Autodesk Fusion 360 part; units mm, degrees
sketch "スケッチ1" plane through (0, 0, 0) normal (0, 1, 0) x (1, 0, 0)
  circle A0 centre (0, 0) radius 14.8
  dimension "d1" = 29.6
extrude "押し出し1" add sketch "スケッチ1" along normal blind 10
sketch "スケッチ2" plane through (0, 10, 0) normal (0, 1, 0) x (-1, 0, 0)
  circle A0 centre (0, 0) radius 14.8
  circle A1 centre (0, 0) radius 16.5
  dimension "d4" = 33
extrude "押し出し2" add sketch "スケッチ2" along normal blind 19 contours A0 | A1
ref_plane "作業平面1" through (0, 24, 0) normal (0, 1, 0) x (-1, 0, 0)
sketch "スケッチ3" plane through (0, 24, 0) normal (0, 1, 0) x (1, 0, 0)
ref_plane "作業平面2" through (0, 29, 0) normal (0, -1, 0) x (-1, 0, 0)
sketch "スケッチ5" plane through (0, 29, 0) normal (0, -1, 0) x (1, 0, 0)
  circle A0 centre (0, 0) radius 19
  dimension "d12" = 38
extrude "押し出し4" add sketch "スケッチ5" against normal blind 2.5
sketch "スケッチ6" plane through (0, 29, 0) normal (0, -1, 0) x (1, 0, 0)
  circle A0 centre (0, 0) radius 18
  dimension "d15" = 36
extrude "押し出し5" add sketch "スケッチ6" along normal blind 2.2
ref_plane "作業平面4" through (0, 24.8, 0) normal (0, -1, 0) x (1, 0, 0)
CAD build for the part. Positions are in the model's coordinates, mm. A direction names the side the tool comes from. Round coordinates to 2 decimals unless told otherwise and drop trailing zeros. Write each loop counter-clockwise with the first axis right and the second up, starting at its lowest first coordinate (ties: lowest second). Pieces come first, ordered by that corner, then holes.
Item 1: Tool access for faces 1 (the cylindrical face through (8.767, 30.232, -16.856)), 2 (the flat face through (8, 26.8, -15)): list every direction of +Z, -Z, +X, -X, +Y, -Y with a clear straight run to the whole face (end or side of a thin tool).
Filled in:
face 1: +Y, -Y
face 2: -Y
Item 2: Band-saw the part on B-B on x = 0. Write the cut outline in (y, z), then the cut area to 3 significant figures.
Filled in:
outline: (0, -14.8) - (10, -14.8) - (10, -16.5) - (26.8, -16.5) - (26.8, -18) - (29, -18) - (29, -19) - (31.5, -19) - (31.5, 19) - (29, 19) - (29, 18) - (26.8, 18) - (26.8, 16.5) - (10, 16.5) - (10, 14.8) - (0, 14.8) - close
area: 1,020 mm2
Item 3: Band-saw the part on C-C on y = 4.5. Write the cut outline in (x, z).
Filled in:
outline: circle Ø29.6 at (0, 0)
Item 4: Drop flat-ended pins along their axis: pin 1 Ø5 at (x, y) = (-11, 4.5) entering from +Z; pin 2 Ø5 at (y, z) = (6, 3.5) entering from +X; pin 3 Ø8 at (y, z) = (13, -10) entering from -X. Give the stop position or say it passes through.
Filled in:
pin 1: stops at z = 12.12
pin 2: stops at x = 14.77
pin 3: stops at x = -15.37
Item 5: Band-saw the part on A-A on z = 0. Write the cut outline in (x, y).
Filled in:
outline: (-19, 29) - (-18, 29) - (-18, 26.8) - (-16.5, 26.8) - (-16.5, 10) - (-14.8, 10) - (-14.8, 0) - (14.8, 0) - (14.8, 10) - (16.5, 10) - (16.5, 26.8) - (18, 26.8) - (18, 29) - (19, 29) - (19, 31.5) - (-19, 31.5) - close
Item 6: Band-saw the part on D-D on y = 13.5. Write the cut outline in (x, z), then the cut area to 3 significant figures.
Filled in:
outline: circle Ø33 at (0, 0)
area: 855 mm2
Item 7: Drill centre lines: L1, parallel to Y at x = 0, z = -15.5; L2, parallel to X at y = 2, z = 0.5; L3, parallel to Y at x = 12, z = 12. Where is each one in solid material? Low to high.
Filled in:
L1: y = 10 to 31.5
L2: x = -14.79 to 14.79
L3: y = 26.8 to 31.5
